The listing builds one solid part. Answer for the finished solid, in the listing's coordinates (mm). Give positions to 0.01 mm unless a question says otherwise; leave off trailing zeros. Write each loop counter-clockwise with the first axis right and the second up, starting at its lowest first coordinate (ties: lowest second). Pieces come first, ordered by that corner, then holes. Notation, with made-up numbers: (-16, 38.25) - (38, 38.25) arc R15 ccw to (38, 66.25) - close; hole circle Ø7 at (-22.75, -15). An arc over 180 degrees is marked (long way). Write each question's results on one line, items separated by ' | '. Start each with the question number.
Q1. Section C-C (x = 151) is taken. Determine the outline of the cut face in (y, z), plus the area to 3 significant figures.
Q2. Section D-D (z = 1.1) is taken. State how many separate pieces and enclosed holes the cut face has, plus the area to 3 significant figures.
Q3. For a pull along X with two mould halves and no side action, classify faces 1 (the face through (-128.982, 118.273, 2.342)), 2 (the face through (-2, 2, 4.75)), 3 (the face through (162.85, 9.24, 2.41)) as pulls with the +X half, pulls with the -X half, needs draft (parallel to the pull), parting line crosses it, or undercut.
Q4. Find the intervals of material crossed by probe 1 along Y at (x, z) = (1, 1.95); probe 2 along X at (y, z) = (-87.25, 1.45); probe 3 along X at (y, z) = (-46.25, 2.4), in increasing order.
Q5. Section A-A (x = 0) is taken. Determine the outline of the cut face in (y, z), plus the area to 3 significant figures.
Q6. Section B-B (y = -12.5) is taken. Determine the outline of the cut face in (x, z).
Q7. Flat-ended cylindrical pins translate along their axes: pin 1 Ø2.5 at (y, z) = (133, 1.5) entering from +X; pin 2 Ø1.4 at (y, z) = (-133.5, 1) entering from -X; pin 3 Ø1 at (y, z) = (66.5, 2) entering from +X. Find the tip coordinate at first contact, or state that the pin passes through.
```python
from build123d import *

# Parameters (mm, degrees)
SKETCH1_R           = 175
BOSS_EXTRUDE1_DEPTH = 4.75
SKETCH2_W           = 80
SKETCH2_H           = 20
SKETCH2_W_2         = 60
SKETCH2_H_2         = 60
CUT_EXTRUDE1_DEPTH  = 4.75
SKETCH3_W           = 10
SKETCH3_H           = 4.75
CUT_EXTRUDE2_DEPTH  = 4.75
SKETCH4_R           = 1.5
CUT_EXTRUDE3_DEPTH  = 248.532952352
SKETCH5_R           = 1.5
CUT_EXTRUDE4_DEPTH  = 248.532952352
SKETCH6_R           = 8.5
CUT_EXTRUDE5_DEPTH  = 4.75
CAVITY1_OUTLINE_R   = 1.5
CAVITY1_DEPTH       = 4.75
SKETCH7_W           = 35
SKETCH7_H           = 160
CUT_EXTRUDE6_DEPTH  = 248.532952352


# Read off the part's stored shape, not the designer's step: Cavity1
with BuildPart() as part:
    # Sketch1 → Boss-Extrude1 (new body)
    with BuildSketch(Plane.XY):
        Circle(SKETCH1_R)
    extrude(amount=BOSS_EXTRUDE1_DEPTH)

    # Sketch2 → Cut-Extrude1 (cut)
    with BuildSketch(Plane(origin=(0, 0, 0), x_dir=(-1, 0, 0), z_dir=(0, 0, -1))):
        with Locations((0, 130)):
            Rectangle(SKETCH2_W, SKETCH2_H)
        with Locations((0, -130)):
            Rectangle(SKETCH2_W, SKETCH2_H)
        with Locations((-100, 0)):
            Rectangle(SKETCH2_W_2, SKETCH2_H_2)
    extrude(amount=-CUT_EXTRUDE1_DEPTH, mode=Mode.SUBTRACT)

    # Sketch3 → Cut-Extrude2 (cut)
    with BuildSketch(Plane.XY.offset(4.75)):
        with Locations((75, 32.375)):
            Rectangle(SKETCH3_W, SKETCH3_H)
        with Locations((125, 32.375)):
            Rectangle(SKETCH3_W, SKETCH3_H)
        with Locations((75, -32.375)):
            Rectangle(SKETCH3_W, SKETCH3_H)
        with Locations((125, -32.375)):
            Rectangle(SKETCH3_W, SKETCH3_H)
    extrude(amount=-CUT_EXTRUDE2_DEPTH, mode=Mode.SUBTRACT)

    # Sketch4 → Cut-Extrude3 (cut, through all)
    with BuildSketch(Plane.XY.offset(4.75)):
        with Locations((-30, -157)):
            Circle(SKETCH4_R)
        with Locations((45, -157)):
            Circle(SKETCH4_R)
        with Locations(Location((-30, 157, 0), (0, 0, 180))):
            Circle(SKETCH4_R)
        with Locations(Location((45, 157, 0), (0, 0, 180))):
            Circle(SKETCH4_R)
        with Locations(Location((45, -93.75, 0), (0, 0, 180))):
            Circle(SKETCH4_R)
        with Locations(Location((-30, -93.75, 0), (0, 0, 180))):
            Circle(SKETCH4_R)
        with Locations((45, 93.75)):
            Circle(SKETCH4_R)
        with Locations((-30, 93.75)):
            Circle(SKETCH4_R)
    extrude(amount=-CUT_EXTRUDE3_DEPTH, mode=Mode.SUBTRACT)

    # Sketch5 → Cut-Extrude4 (cut, through all)
    with BuildSketch(Plane.XY.offset(4.75)):
        with Locations((89.5, 87.25)):
            Circle(SKETCH5_R)
        with Locations((130.5, 87.25)):
            Circle(SKETCH5_R)
        with Locations((130.5, 46.25)):
            Circle(SKETCH5_R)
        with Locations((89.5, 46.25)):
            Circle(SKETCH5_R)
        with Locations(Location((89.5, -87.25, 0), (0, 0, 180))):
            Circle(SKETCH5_R)
        with Locations(Location((130.5, -87.25, 0), (0, 0, 180))):
            Circle(SKETCH5_R)
        with Locations(Location((130.5, -46.25, 0), (0, 0, 180))):
            Circle(SKETCH5_R)
        with Locations(Location((89.5, -46.25, 0), (0, 0, 180))):
            Circle(SKETCH5_R)
    extrude(amount=-CUT_EXTRUDE4_DEPTH, mode=Mode.SUBTRACT)

    # Sketch6 → Cut-Extrude5 (cut)
    with BuildSketch(Plane.XY.offset(4.75)):
        with Locations((155, 12.5)):
            Circle(SKETCH6_R)
        with Locations((155, -12.5)):
            Circle(SKETCH6_R)
    extrude(amount=-CUT_EXTRUDE5_DEPTH, mode=Mode.SUBTRACT)

    # Cavity1 outline → Cavity1 (cut)
    with BuildSketch(Plane.XY):
        with Locations((72.337603572, -125.375)):
            Circle(CAVITY1_OUTLINE_R)
        with Locations((72.337603572, 125.375)):
            Circle(CAVITY1_OUTLINE_R)
    extrude(amount=CAVITY1_DEPTH, mode=Mode.SUBTRACT)

    # Sketch7 → Cut-Extrude6 (cut, through all)
    with BuildSketch(Plane.XY.offset(4.75)):
        with Locations((42.5, 0)):
            Rectangle(SKETCH7_W, SKETCH7_H)
    extrude(amount=-CUT_EXTRUDE6_DEPTH, mode=Mode.SUBTRACT)


solid = part.part
```
Answers below:
1) outline: (-88.45, 0) - (-20, 0) - (-20, 4.75) - (-88.45, 4.75) - close; (-5, 0) - (5, 0) - (5, 4.75) - (-5, 4.75) - close; (20, 0) - (88.45, 0) - (88.45, 4.75) - (20, 4.75) - close | area: 698 mm2
2) separate pieces: 1 | enclosed holes: 24 | area: 83,000 mm2
3) face 1: parting line crosses it | face 2: needs draft | face 3: undercut
4) probe 1: y = -175 to -140, -120 to 120, 140 to 175 | probe 2: x = -151.7 to 88, 91 to 129, 132 to 151.7 | probe 3: x = -168.78 to 25, 60 to 88, 91 to 129, 132 to 168.78
5) outline: (-175, 0) - (-140, 0) - (-140, 4.75) - (-175, 4.75) - close; (-120, 0) - (120, 0) - (120, 4.75) - (-120, 4.75) - close; (140, 0) - (175, 0) - (175, 4.75) - (140, 4.75) - close | area: 1,470 mm2
6) outline: (-174.55, 0) - (25, 0) - (25, 4.75) - (-174.55, 4.75) - close; (60, 0) - (70, 0) - (70, 4.75) - (60, 4.75) - close; (130, 0) - (146.5, 0) - (146.5, 4.75) - (130, 4.75) - close; (163.5, 0) - (174.55, 0) - (174.55, 4.75) - (163.5, 4.75) - close
7) pin 1: stops at x = 115.18 | pin 2: stops at x = -113.97 | pin 3: stops at x = 162.08
